Design review of the part built by this model. Coordinates are the model's own, in mm. Round coordinates to 2 decimals unless told otherwise and drop trailing zeros. Order: outer loops, then holes, each group sorted by start corner. A loop starts at its lowest first (then second) coordinate and runs counter-clockwise, first axis right, second up. Notation, with made-up numbers: (-18.5, -26) - (33.5, -26) arc R6 ccw to (33.5, -19) - close; hole circle Ø6 at (72.5, -32). An arc over 180 degrees is marked (long way). Write item = value, one per line.
from build123d import *

# Parameters (mm, degrees)
SKETCH1_W           = 254
SKETCH1_H           = 228.6
BOSS_EXTRUDE1_DEPTH = 4.826
CUT_EXTRUDE3_DEPTH  = 4.826
SKETCH19_W          = 4.826
SKETCH19_H          = 8.466666666
CUT_EXTRUDE16_DEPTH = 171.929167423
FILLET11_R          = 50.8
SKETCH20_W          = 10.16
SKETCH20_H          = 63.5
CUT_EXTRUDE17_DEPTH = 171.929167423
SKETCH23_R          = 1.905
CUT_EXTRUDE18_DEPTH = 171.929167423
SKETCH24_W          = 20.32
SKETCH24_H          = 4.826
CUT_EXTRUDE19_DEPTH = 171.929167423
SKETCH26_R          = 24.13
CUT_EXTRUDE20_DEPTH = 171.929167423
SKETCH27_W          = 4.826
SKETCH27_H          = 12.7
CUT_EXTRUDE21_DEPTH = 171.929167423
SKETCH28_R          = 19.05
CUT_EXTRUDE22_DEPTH = 171.929167423


with BuildPart() as part:
    # Sketch1 → Boss-Extrude1 (new body)
    with BuildSketch(Plane(origin=(0, 0, 0), x_dir=(1, 0, 0), z_dir=(0, 1, 0))):
        Rectangle(SKETCH1_W, SKETCH1_H)
    extrude(amount=BOSS_EXTRUDE1_DEPTH)

    # Sketch4 → Cut-Extrude3 (cut)
    with BuildSketch(Plane(origin=(0, 4.826, 0), x_dir=(1, 0, 0), z_dir=(0, 1, 0))):
        with BuildLine():
            Line((-127, 88.9), (-127, 114.3))
            Line((-127, 114.3), (-101.6, 114.3))
            ThreePointArc((-101.6, 114.3), (-119.560512242, 106.860512242), (-127, 88.9))
        make_face()
        with BuildLine():
            Line((127, 88.9), (127, 114.3))
            Line((127, 114.3), (101.6, 114.3))
            ThreePointArc((101.6, 114.3), (119.560512242, 106.860512242), (127, 88.9))
        make_face()
    extrude(amount=-CUT_EXTRUDE3_DEPTH, mode=Mode.SUBTRACT)

    # Sketch19 → Cut-Extrude16 (cut, through all)
    with BuildSketch(Plane(origin=(0, 4.826, 0), x_dir=(1, 0, 0), z_dir=(0, 1, 0))):
        with Locations((-98.58699993, -34.925)):
            Rectangle(SKETCH19_W, SKETCH19_H)
        with Locations((-98.58699993, 53.975)):
            Rectangle(SKETCH19_W, SKETCH19_H)
    extrude(amount=-CUT_EXTRUDE16_DEPTH, mode=Mode.SUBTRACT)

    # Fillet11
    fillet11_edges = [part.edges().sort_by_distance(p)[0] for p in [
        (127, 2.413, 114.3),
        (-127, 2.413, 114.3),
    ]]
    fillet(fillet11_edges, radius=FILLET11_R)

    # Sketch20 → Cut-Extrude17 (cut, through all)
    with BuildSketch(Plane.XZ):
        with Locations((106.07999993, 34.925)):
            Rectangle(SKETCH20_W, SKETCH20_H)
    extrude(amount=-CUT_EXTRUDE17_DEPTH, mode=Mode.SUBTRACT)

    # Sketch23 → Cut-Extrude18 (cut, through all)
    with BuildSketch(Plane(origin=(0, 4.826, 0), x_dir=(1, 0, 0), z_dir=(0, 1, 0))):
        with Locations(Location((70.741119647, -25.576370111, 0), (0, 0, 270))):
            Circle(SKETCH23_R)
        with Locations(Location((70.741119647, -66.216370111, 0), (0, 0, 270))):
            Circle(SKETCH23_R)
        with Locations(Location((19.941119647, -25.576370111, 0), (0, 0, 270))):
            Circle(SKETCH23_R)
        with Locations(Location((19.941119647, -66.216370111, 0), (0, 0, 270))):
            Circle(SKETCH23_R)
        with Locations(Location((-11.48044922, 5.792629889, 0), (0, 0, 270))):
            Circle(SKETCH23_R)
        with Locations(Location((-64.82044922, 5.792629889, 0), (0, 0, 270))):
            Circle(SKETCH23_R)
        with Locations(Location((-64.82044922, -66.851370111, 0), (0, 0, 270))):
            Circle(SKETCH23_R)
        with Locations(Location((-11.48044922, -66.851370111, 0), (0, 0, 270))):
            Circle(SKETCH23_R)
    extrude(amount=-CUT_EXTRUDE18_DEPTH, mode=Mode.SUBTRACT)

    # Sketch24 → Cut-Extrude19 (cut, through all)
    with BuildSketch(Plane.XZ):
        with Locations((40.64, 111.887)):
            Rectangle(SKETCH24_W, SKETCH24_H)
        with Locations((-40.64, 111.887)):
            Rectangle(SKETCH24_W, SKETCH24_H)
        with Locations((0, 111.887)):
            Rectangle(SKETCH24_W, SKETCH24_H)
    extrude(amount=-CUT_EXTRUDE19_DEPTH, mode=Mode.SUBTRACT)

    # Sketch26 → Cut-Extrude20 (cut, through all)
    with BuildSketch(Plane.XZ):
        with Locations(Location((0, -55.982011538, 0), (0, 0, 270))):
            Circle(SKETCH26_R)
    extrude(amount=-CUT_EXTRUDE20_DEPTH, mode=Mode.SUBTRACT)

    # Sketch27 → Cut-Extrude21 (cut, through all)
    with BuildSketch(Plane.XZ):
        with Locations((-48.387, 90.424)):
            Rectangle(SKETCH27_W, SKETCH27_H)
        with Locations((48.387, 90.424)):
            Rectangle(SKETCH27_W, SKETCH27_H)
    extrude(amount=-CUT_EXTRUDE21_DEPTH, mode=Mode.SUBTRACT)

    # Sketch28 → Cut-Extrude22 (cut, through all)
    with BuildSketch(Plane(origin=(0, 4.826, 0), x_dir=(1, 0, 0), z_dir=(0, 1, 0))):
        with Locations(Location((45.341119647, 0, 0), (0, 0, 270))):
            Circle(SKETCH28_R)
    extrude(amount=-CUT_EXTRUDE22_DEPTH, mode=Mode.SUBTRACT)


solid = part.part
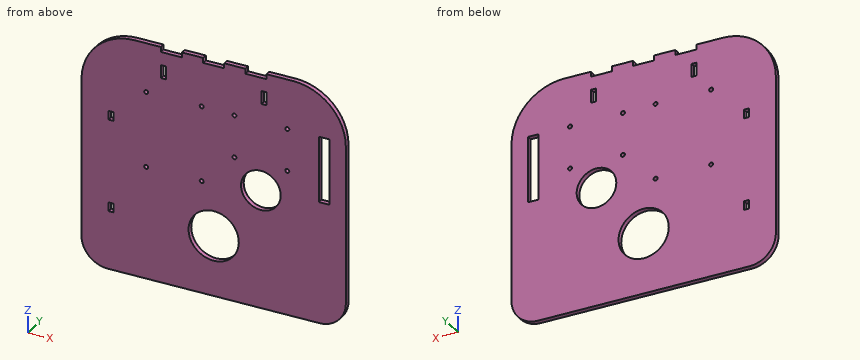
Item 1: Take a section at B-B, the plane z = 0. State the section outline as (x, y) points, and give its area (3 significant figures).
Data:
outline = (-127, 0) - (26.29, 0) - (26.29, 4.83) - (-127, 4.83) - close; (64.39, 0) - (127, 0) - (127, 4.83) - (64.39, 4.83) - close
area = 1,040 mm2
Item 2: Insertion check: P1, Ø2.5, axis at y = 3, z = 111, coming from the +X side; P2, Ø1.4, axis at y = 3, z = 111, coming from the -X side; P3, Ø1, axis at x = 90.5, y = 2.5, coming from the +Z side. Each pin has a flat end and moves straight along its axis. Give the tip position at first contact, or say it passes through.
Data:
P1 = 97.21
P2 = -95.96
P3 = 112.39
Item 3: Take a section at C-C, the plane y = 3.35. Count the separate pieces of the cut face and the enclosed holes in it, and give its area (3 significant figures).
Data:
separate_pieces = 1
enclosed_holes = 15
area = 52,500 mm2
Item 4: Take a section at A-A, the plane x = 0. State the section outline as (y, z) points, and give its area (3 significant figures).
Data:
outline = (0, -114.3) - (4.83, -114.3) - (4.83, -80.11) - (0, -80.11) - close; (0, -31.85) - (4.83, -31.85) - (4.83, 109.47) - (0, 109.47) - close
area = 847 mm2
Item 5: For line 1 along X through (y, z) = (2.05, -57); line 2 along X through (y, z) = (2, 48); line 3 along Z through (x, y) = (20, 2.7), list the stretches that pass through material, from the lowest coordinate up. Write a range as [from, to].
Data:
line_1 = [-127, -101], [-96.17, -24.11], [24.11, 127]
line_2 = [-127, 101], [111.16, 127]
line_3 = [-114.3, -69.48], [-42.48, 23.67], [27.48, 64.31], [68.12, 114.3]
